Here's how the part is built. I have some questions about the finished solid (model axes, mm). A direction names the side the tool comes from. Give positions to 0.01 mm unless a question says otherwise; leave off trailing zeros. Order: outer loops, then holes, each group sorted by start corner. A loop starts at its lowest first (then second) coordinate and runs counter-clockwise, first axis right, second up. Notation, with made-up numbers: (59.25, -25) -> (84.25, -25) arc R30 ccw to (84.25, -2) -> close; hole circle Ø8 at (56, 82.5). An arc over 180 degrees is marked (long way). Write each question's results on one line, items separated by ' | '. Start each with the question number.
Q1. Thinking about a two-plate mould opening in Y: for faces 5 (the face through (-15.41, 9.86, 0.78)), 6 (the face through (-4, 4, 0)), 7 (the face through (-13.606, 12.147, 0.783)), 8 (the face through (-15.51, 12.125, 0.783)), which applies, pulls with the +Y half, pulls with the -Y half, needs draft (parallel to the pull), parting line crosses it, or undercut?
Q2. Imagine slicing it at B-B, the plane y = 0. Please give me the cut outline in (x, z), then the cut area to 3 significant figures.
Q3. Imagine slicing it at A-A, the plane x = -12.5. Please give me the cut outline in (y, z), then the cut area to 3 significant figures.
Q4. I need wall thicknesses on line 1 along X through (y, z) = (12.75, 0.3); line 2 along X through (y, z) = (8.75, 1.5); line 3 along Y through (x, z) = (0, 0.4). Which ranges of each line are inside material? Lowest first, please. Write a range as [from, to].
Q5. For faces 1 (the face through (15.524, 12.111, 0.783)), 2 (the face through (2.965, 1.118, 0.783)), 3 (the face through (9.535, 10.016, 0.783)), 4 (the face through (15.4, 9.85, 0.78)), which set-ups out of +Z, -Z, +X, -X, +Y, -Y let a thin tool reach every point of the face, with its end or its side?
Q6. Imagine slicing it at D-D, the plane x = 4.5. Please give me the cut outline in (y, z), then the cut area to 3 significant figures.
Q7. I'm going to push flat-ended pins straight in: pin 1 (5 mm diameter, centred on x = -12.5, y = 11.13, fed in from -Z); pin 2 (3 mm diameter, centred on x = 7.5, y = 1, fed in from +Z). Where does each tip first touch, or does it pass through?
Q8. Imagine slicing it at C-C, the plane z = 0.7. State how many separate pieces and enclosed holes the cut face has, then the cut area to 3 significant figures.
```python
from build123d import *

# Parameters (mm, degrees)
SKETCH4_R           = 1.5
SKETCH4_R_2         = 1.500000001
SKETCH4_R_3         = 1.499999998
BOSS_EXTRUDE2_DEPTH = 1.5875


with BuildPart() as part:
    # Sketch4 → Boss-Extrude2 (new body)
    with BuildSketch(Plane.XY):
        with BuildLine():
            Line((-1.921662056, 3.050772843), (-9.248103317, 9.576404551))
            ThreePointArc((-9.248103317, 9.576404551), (-9.532363934, 10.009007248), (-9.562239502, 10.525782482))
            ThreePointArc((-9.562239502, 10.525782482), (-11.501295907, 13.962584592), (-15.168282223, 12.504928996))
            ThreePointArc((-15.168282223, 12.504928996), (-15.515981129, 12.121451925), (-16.008835749, 11.963200494))
            Line((-16.008835749, 11.963200494), (-16.599403965, 11.934302598))
            ThreePointArc((-16.599403965, 11.934302598), (-17.103207742, 12.042580302), (-17.486208385, 12.387330667))
            ThreePointArc((-17.486208385, 12.387330667), (-22.995673813, 10.588945924), (-17.32515244, 9.391622098))
            ThreePointArc((-17.32515244, 9.391622098), (-16.977285242, 9.77807758), (-16.482410468, 9.937634422))
            Line((-16.482410468, 9.937634422), (-15.911087986, 9.965590578))
            ThreePointArc((-15.911087986, 9.965590578), (-15.405137648, 9.856213028), (-15.021660578, 9.508514122))
            ThreePointArc((-15.021660578, 9.508514122), (-13.498704093, 8.304814666), (-11.557591443, 8.285565834))
            ThreePointArc((-11.557591443, 8.285565834), (-11.040816209, 8.315441402), (-10.578337944, 8.082926785))
            Line((-10.578337944, 8.082926785), (-3.251896683, 1.557295078))
            ThreePointArc((-3.251896683, 1.557295078), (-2.967636066, 1.124692381), (-2.937760498, 0.607917146))
            ThreePointArc((-2.937760498, 0.607917146), (0, -3), (2.937760498, 0.607917146))
            ThreePointArc((2.937760498, 0.607917146), (2.967636066, 1.124692381), (3.251896683, 1.557295078))
            Line((3.251896683, 1.557295078), (10.578337944, 8.082926785))
            ThreePointArc((10.578337944, 8.082926785), (11.040816209, 8.315441402), (11.557591443, 8.285565834))
            ThreePointArc((11.557591443, 8.285565834), (13.495560549, 8.303706839), (15.01804315, 9.502914943))
            ThreePointArc((15.01804315, 9.502914943), (15.40229187, 9.849760895), (15.908483998, 9.958013941))
            Line((15.908483998, 9.958013941), (16.48932974, 9.928297901))
            ThreePointArc((16.48932974, 9.928297901), (16.981831505, 9.768951725), (17.328677456, 9.384703006))
            ThreePointArc((17.328677456, 9.384703006), (22.996081677, 10.596720608), (17.481956847, 12.380784685))
            ThreePointArc((17.481956847, 12.380784685), (17.097708128, 12.033938733), (16.591516, 11.925685687))
            Line((16.591516, 11.925685687), (16.010670258, 11.955401727))
            ThreePointArc((16.010670258, 11.955401727), (15.518168493, 12.114747903), (15.171322541, 12.498996622))
            ThreePointArc((15.171322541, 12.498996622), (11.504439451, 13.963692419), (9.562239502, 10.525782482))
            ThreePointArc((9.562239502, 10.525782482), (9.532363934, 10.009007248), (9.248103317, 9.576404551))
            Line((9.248103317, 9.576404551), (1.921662056, 3.050772843))
            ThreePointArc((1.921662056, 3.050772843), (1.459183791, 2.818258227), (0.942408557, 2.848133795))
            ThreePointArc((0.942408557, 2.848133795), (0, 3), (-0.942408557, 2.848133795))
            ThreePointArc((-0.942408557, 2.848133795), (-1.459183791, 2.818258227), (-1.921662056, 3.050772843))
        make_face()
        with Locations((-12.5, 11.133699629)):
            Circle(SKETCH4_R, mode=Mode.SUBTRACT)
        with Locations((-20.000000001, 10.750000001)):
            Circle(SKETCH4_R_2, mode=Mode.SUBTRACT)
        Circle(SKETCH4_R, mode=Mode.SUBTRACT)
        with Locations((12.5, 11.133699629)):
            Circle(SKETCH4_R, mode=Mode.SUBTRACT)
        with Locations((19.999999998, 10.749999999)):
            Circle(SKETCH4_R_3, mode=Mode.SUBTRACT)
    extrude(amount=BOSS_EXTRUDE2_DEPTH)


solid = part.part
```
Geometry check:
1) face 5: pulls with the -Y half | face 6: needs draft | face 7: undercut | face 8: pulls with the +Y half
2) outline: (-3, 0) -> (-1.5, 0) -> (-1.5, 1.59) -> (-3, 1.59) -> close; (1.5, 0) -> (3, 0) -> (3, 1.59) -> (1.5, 1.59) -> close | area: 4.76 mm²
3) outline: (8.13, 0) -> (9.63, 0) -> (9.63, 1.59) -> (8.13, 1.59) -> close; (12.63, 0) -> (14.13, 0) -> (14.13, 1.59) -> (12.63, 1.59) -> close | area: 4.76 mm²
4) line 1: [-22.24, -17.76], [-15.03, -9.97], [9.97, 15.03], [17.76, 22.24] | line 2: [-22.24, -17.76], [-14.32, -8.32], [8.32, 14.32], [17.76, 22.24] | line 3: [-3, -1.5], [1.5, 3]
5) face 1: +Z, -Z, +Y | face 2: +Z, -Z, +X | face 3: +Z, -Z | face 4: +Z, -Z, -Y
6) outline: (2.67, 0) -> (5.35, 0) -> (5.35, 1.59) -> (2.67, 1.59) -> close | area: 4.25 mm²
7) pin 1: z = 0 | pin 2: through
8) separate pieces: 1 | enclosed holes: 5 | area: 157 mm²
